Check sheet for the modelled part. Datum: model origin and axes. Units: mm. A direction names the side the tool comes from. Give positions to 0.01 mm unless a question says otherwise; leave off trailing zeros. Order: outer loops, then holes, each group sorted by start corner. A loop starts at its lowest first (then second) coordinate and runs counter-clockwise, first axis right, second up. Notation, with made-up numbers: M 52,59.25 L 93,59.25 A29 ccw 93,89.25 Z; hole C 59.25,-9.5 d9. An arc over 180 degrees is marked long. Return JSON: item names as keys, results as strings. Group by question number.
from build123d import *

# Parameters (mm, degrees)
SKETCH1_R           = 18.161
BOSS_EXTRUDE1_DEPTH = 26.543
SKETCH2_R           = 16.51
BOSS_EXTRUDE2_DEPTH = 22.606
SKETCH3_R           = 4.5085
BOSS_EXTRUDE3_DEPTH = 3.302
SKETCH4_R           = 2.413
BOSS_EXTRUDE4_DEPTH = 1.27
SKETCH5_R           = 5.969
BOSS_EXTRUDE5_DEPTH = 4.3688
BOSS_EXTRUDE6_DEPTH = 15.24
SKETCH8_W           = 5.588
SKETCH8_H           = 2.794
SKETCH8_R           = 0.635
BOSS_EXTRUDE7_DEPTH = 0.254
CIRPATTERN1_COUNT   = 2
CIRPATTERN2_COUNT   = 12


with BuildPart() as part:
    # Sketch1 → Boss-Extrude1 (new body)
    with BuildSketch(Plane.XY):
        Circle(SKETCH1_R)
    extrude(amount=BOSS_EXTRUDE1_DEPTH)

    # Sketch2 → Boss-Extrude2 (add)
    with BuildSketch(Plane(origin=(0, 0, 0), x_dir=(-1, 0, 0), z_dir=(0, 0, -1))):
        Circle(SKETCH2_R)
    extrude(amount=BOSS_EXTRUDE2_DEPTH)

    # Sketch3 → Boss-Extrude3 (add)
    with BuildSketch(Plane(origin=(0, 0, -22.606), x_dir=(-1, 0, 0), z_dir=(0, 0, -1))):
        Circle(SKETCH3_R)
    extrude(amount=BOSS_EXTRUDE3_DEPTH)

    # Sketch4 → Boss-Extrude4 (add)
    with BuildSketch(Plane(origin=(0, 0, -22.606), x_dir=(-1, 0, 0), z_dir=(0, 0, -1))):
        with Locations((0, -12.7)):
            Circle(SKETCH4_R)
        with Locations((0, 12.7)):
            Circle(SKETCH4_R)
    extrude(amount=BOSS_EXTRUDE4_DEPTH)

    # Sketch5 → Boss-Extrude5 (add)
    with BuildSketch(Plane.XY.offset(26.543)):
        with Locations((0, -7.366)):
            Circle(SKETCH5_R)
    extrude(amount=BOSS_EXTRUDE5_DEPTH)

    # Sketch6 → Boss-Extrude6 (add)
    with BuildSketch(Plane.XY.offset(30.9118)):
        with BuildLine():
            Line((-1.715657017, -4.905), (1.715657017, -4.905))
            ThreePointArc((1.715657017, -4.905), (0, -10.366), (-1.715657017, -4.905))
        make_face()
    extrude(amount=BOSS_EXTRUDE6_DEPTH)

    # Sketch8 → Boss-Extrude7 (add, symmetric)
    with BuildSketch(Plane.ZX.offset(12.7)):
        with Locations((-26.67, 0)):
            Rectangle(SKETCH8_W, SKETCH8_H)
        with Locations((-28.067, 0)):
            Circle(SKETCH8_R, mode=Mode.SUBTRACT)
    boss_extrude7 = extrude(amount=BOSS_EXTRUDE7_DEPTH, both=True)

    # CirPattern1: Boss-Extrude7 ×2 about axis
    cirpattern1_axis = Axis((0, 0, 0), (0, 0, 1))
    for i in range(1, CIRPATTERN1_COUNT):
        add(boss_extrude7.rotate(cirpattern1_axis, i * 360 / CIRPATTERN1_COUNT))

    # Sketch12 → 3.0mm Dowel Hole1 (revolve, cut)
    with BuildSketch(Plane(origin=(0, 15.494, 26.543), x_dir=(0, -1, 0), z_dir=(1, 0, 0))):
        Polygon((0, 0), (0, 11.061290929), (1.5, 10.16), (1.5, 0), align=None)
    f_3_0mm_dowel_hole1 = revolve(axis=Axis((0, 15.494, 32.893), (0, 0, -1)), mode=Mode.SUBTRACT)

    # CirPattern2: 3.0mm Dowel Hole1 ×12 about axis, 5 skipped
    cirpattern2_axis = Axis((0, 0, 26.543), (0, 0, -1))
    add([f_3_0mm_dowel_hole1.rotate(cirpattern2_axis, i * 360 / CIRPATTERN2_COUNT) for i in range(1, CIRPATTERN2_COUNT) if i not in (1, 2, 5, 6, 10)], mode=Mode.SUBTRACT)


solid = part.part
1) Material ranges on line 1 along Y through (x, z) = (-7, 26); line 2 along Z through (x, y) = (5, -1); line 3 along Z through (x, y) = (0, 12), recorded low to high.
2) Depth check by flat-ended pin: P1, Ø2.5, axis at x = -7.75, y = 13.42, coming from the -Z side; P2, Ø3, axis at x = 0.5, z = -28, coming from the -Y side; P3, Ø3, axis at x = 1, z = 29, coming from the -Y side (3 decimals); P4, Ø0.8, axis at x = 0, z = -28.067, coming from the +Y side. Enter the tip coordinate at first touch or a pass-through.
3) Sectioned sample at C-C on z = -17.5. Record the boundary of the cut face in (x, y).
4) Sectioned sample at B-B on y = 9. Record the boundary of the cut face in (x, z).
5) Sectioned sample at A-A on z = 22.5. Record the boundary of the cut face in (x, y), then the cut area to 3 significant figures.
6) Tool access check on faces 1 (the face through (-3.4, -3.4, -22.606)), 2 (the face through (0, 0, -25.908)), 3 (the face through (0, -4.905, 38)), 4 (the face through (14.75, -8.44, 21.53)). Record the directions out of +Z, -Z, +X, -X, +Y, -Y that give a thin tool (end or side, any length) a straight path to the whole face; none if there is none.
7) Release check for a two-part mould opening along Y. For faces 5 (the face through (0, -12.954, -27)), 6 (the face through (8, -15, 0)), 7 (the face through (-0.066, 16.993, 21.534)), 8 (the face through (-16.993, -0.066, 21.534)) record: released by +Y, released by -Y, zero draft, split by the parting line, or undercut.
Reply:
{
 "1": {"line 1": "-16.76 to -14.72, -12.12 to 12.12, 14.72 to 16.76", "line 2": "-22.61 to 26.54", "line 3": "-23.88 to 26.54"},
 "2": {"P1": "z = -22.61", "P2": "y = -12.95", "P3": "y = -13.335", "P4": "through"},
 "3": {"outline": "C 0,0 d33.02"},
 "4": {"outline": "M -15.77,0 L -13.84,0 L -13.84,-22.61 L 13.84,-22.61 L 13.84,0 L 15.77,0 L 15.77,26.54 L -15.77,26.54 Z"},
 "5": {"outline": "C 0,0 d36.32; hole C -15.49,0 d3; hole C -13.42,-7.75 d3; hole C -7.75,-13.42 d3; hole C -7.75,13.42 d3; hole C 0,15.49 d3; hole C 13.42,-7.75 d3; hole C 15.49,0 d3", "area": "987 mm^2"},
 "6": {"face 1": "-Z", "face 2": "-Z, +X, -X", "face 3": "+Z, +X, -X, +Y", "face 4": "+Z"},
 "7": {"face 5": "released by -Y", "face 6": "zero draft", "face 7": "undercut", "face 8": "undercut"}
}
